```python
from build123d import *

# Parameters (mm, degrees)
SKETCH1_W           = 150
SKETCH1_H           = 95
BOSS_EXTRUDE1_DEPTH = 5
SKETCH2_W           = 145
SKETCH2_H           = 85
BOSS_EXTRUDE2_DEPTH = 3.75
SKETCH3_W           = 145
SKETCH3_H           = 90
BOSS_EXTRUDE3_DEPTH = 2.5
FILLET2_R           = 2.5


with BuildPart() as part:
    # Sketch1 → Boss-Extrude1 (new body)
    with BuildSketch(Plane(origin=(0, 0, 0), x_dir=(1, 0, 0), z_dir=(0, 1, 0))):
        with Locations((75, 47.5)):
            Rectangle(SKETCH1_W, SKETCH1_H)
    extrude(amount=BOSS_EXTRUDE1_DEPTH)

    # Sketch2 → Boss-Extrude2 (add)
    with BuildSketch(Plane(origin=(0, 5, 0), x_dir=(1, 0, 0), z_dir=(0, 1, 0))):
        with Locations((77.5, 47.5)):
            Rectangle(SKETCH2_W, SKETCH2_H)
    extrude(amount=BOSS_EXTRUDE2_DEPTH)

    # Sketch3 → Boss-Extrude3 (add)
    with BuildSketch(Plane(origin=(0, 8.75, 0), x_dir=(1, 0, 0), z_dir=(0, 1, 0))):
        with Locations((77.5, 47.5)):
            Rectangle(SKETCH3_W, SKETCH3_H)
    extrude(amount=BOSS_EXTRUDE3_DEPTH)

    # Fillet2
    fillet2_edges = [part.edges().sort_by_distance(p)[0] for p in [
        (0, 2.5, -95),
        (150, 2.5, -95),
        (150, 2.5, 0),
        (0, 2.5, 0),
    ]]
    fillet(fillet2_edges, radius=FILLET2_R)


solid = part.part
```
Check sheet for the modelled part. Datum: model origin and axes. Units: mm. A direction names the side the tool comes from. Round coordinates to 2 decimals unless told otherwise and drop trailing zeros. Order: outer loops, then holes, each group sorted by start corner. A loop starts at its lowest first (then second) coordinate and runs counter-clockwise, first axis right, second up. Notation, with made-up numbers: (28.25, 54.5) -> (73.25, 54.5) arc R14 ccw to (73.25, 62.5) -> close; hole circle Ø6 at (44, -17). An arc over 180 degrees is marked (long way). One line per item, written item: value. Start each with the question number.
Q1. Thickness scan on line 1 (X direction, y = 10.5, z = -7.5); line 2 (Z direction, x = 136.5, y = 5.75); line 3 (Z direction, x = 134, y = 9.25). Record the ranges inside material, lowest first.
Q2. Set-up check for faces 1 (the face through (74, 2, -95)), 2 (the face through (5, 8, -47)): record each of +Z, -Z, +X, -X, +Y, -Y from which the full face is reachable in a straight line by a thin tool's end or side.
Q3. Gauge pin test, flat ends, axial feed: pin 1 Ø3 at (x, y) = (78.5, 7) entering from -Z; pin 2 Ø1.1 at (x, y) = (65.5, 6) entering from +Z; pin 3 Ø0.8 at (x, y) = (87, 10) entering from +Z. Record the tip position at first contact, or that the pin passes through.
Q4. Cross-section at C-C (y = 6.5). Record the boundary of the cut face in (x, z).
Q5. Cross-section at A-A (x = 91). Record the boundary of the cut face in (y, z).
Q6. Mould release check, pull along Y, two halves, no side actions. Record for faces 3 (the face through (76, 7, -90)), 4 (the face through (76, 7, -5)), 5 (the face through (76, 11.25, -48)), 6 (the face through (0, 2, -47)): pulls with the +Y half, pulls with the -Y half, needs draft (parallel to the pull), parting line crosses it, or undercut.
Q7. Cross-section at B-B (z = -42.5). Record the boundary of the cut face in (x, y), and give its area (3 significant figures).
Completed:
1. line 1: x = 5 to 150
1. line 2: z = -90 to -5
1. line 3: z = -92.5 to -2.5
2. face 1: -Z, +X, -X, +Y, -Y
2. face 2: +Z, -Z, -X, +Y
3. pin 1: stops at z = -90
3. pin 2: stops at z = -5
3. pin 3: stops at z = -2.5
4. outline: (5, -90) -> (150, -90) -> (150, -5) -> (5, -5) -> close
5. outline: (0, -95) -> (5, -95) -> (5, -90) -> (8.75, -90) -> (8.75, -92.5) -> (11.25, -92.5) -> (11.25, -2.5) -> (8.75, -2.5) -> (8.75, -5) -> (5, -5) -> (5, 0) -> (0, 0) -> close
6. face 3: undercut
6. face 4: undercut
6. face 5: pulls with the +Y half
6. face 6: needs draft
7. outline: (0, 0) -> (150, 0) -> (150, 11.25) -> (5, 11.25) -> (5, 5) -> (0, 5) -> close
7. area: 1,660 mm²
